```python
from build123d import *

# Parameters (mm, degrees)
SKETCH1_W           = 109.238
SKETCH1_H           = 62.54
BOSS_EXTRUDE1_DEPTH = 3
SKETCH2_W           = 107.238
SKETCH2_H           = 60.54
SKETCH2_W_2         = 105.238
SKETCH2_H_2         = 58.54
BOSS_EXTRUDE2_DEPTH = 3
BOSS_EXTRUDE2_TAPER = 45


with BuildPart() as part:
    # Sketch1 → Boss-Extrude1 (new body)
    with BuildSketch(Plane(origin=(0, 0, 0), x_dir=(1, 0, 0), z_dir=(0, 1, 0))):
        Rectangle(SKETCH1_W, SKETCH1_H)
    extrude(amount=BOSS_EXTRUDE1_DEPTH)

    # Sketch2 → Boss-Extrude2 (add)
    with BuildSketch(Plane.XZ):
        Rectangle(SKETCH2_W, SKETCH2_H)
        Rectangle(SKETCH2_W_2, SKETCH2_H_2, mode=Mode.SUBTRACT)
    extrude(amount=BOSS_EXTRUDE2_DEPTH, taper=BOSS_EXTRUDE2_TAPER)


solid = part.part
```
Source: CAD feature listing. Evaluate the final solid. Frame: model axes, mm. Round coordinates to 2 decimals unless told otherwise and drop trailing zeros. Use a Markdown table: item, result. Add a question column.
1. Pull-direction query (X, two-part tool) for faces 1 (the flat face through (-1, 1, -31.27)), 2 (the flat face through (54.619, 1, 0)), 3 (the flat face through (-1, 0, 0)); classes: +X half, -X half, draft (parallel to the pull), parting line (faces both ways), or undercut.
2. Contact query for flat-ended pins moving along their axis: pin 1 (12 mm diameter, centred on x = 33.5, z = -25, fed in from -Y); pin 2 (3 mm diameter, centred on x = 4, z = 3, fed in from -Y). Output: stop coordinate, or through.
3. Ray query, line 1 along Y through (x, z) = (-22, 25); line 2 along Z through (x, y) = (29, -0.15); line 3 along Z through (x, y) = (-11, -0.1). Return the intervals inside material, ascending. Write a range as [from, to].
Solution:
| question | item | result |
|---|---|---|
| 1 | face 1 | draft |
| 1 | face 2 | +X half |
| 1 | face 3 | undercut |
| 2 | pin 1 | stops at y = -0.5 |
| 2 | pin 2 | stops at y = 0 |
| 3 | line 1 | y = [0, 3] |
| 3 | line 2 | z = [-30.12, -29.42], [29.42, 30.12] |
| 3 | line 3 | z = [-30.17, -29.37], [29.37, 30.17] |
